Check sheet for the drawn part. Datum: minimum x, y, z corner. Units: mm. A direction names the side the tool comes from. Give positions to 0.01 mm unless a question says otherwise; leave off trailing zeros. Order: outer loops, then holes, each group sorted by start corner. A loop starts at its lowest first (then second) coordinate and runs counter-clockwise, first axis right, second up. Notation, with made-up numbers: M 84.5,16 L 119.5,16 A24 cw 119.5,27 Z; hole C 65,55.5 d11. An arc over 180 degrees is marked long. Answer as CSV lines item,"result". Start each with the question number.
Q1. Set-up check for the marked faces 1 and 2: record each of +Z, -Z, +X, -X, +Y, -Y from which the full face is reachable in a straight line by a thin tool's end or side.
Q2. Section check C-C, the plane z = 3.5. Record the boundary of the cut face in (x, y), then the cut area to 3 significant figures.
Q3. Go/stop test with flat-tipped pins: pin 1 (1.5 mm diameter, centred on y = 5.5, z = 3, fed in from +X); pin 2 (2.5 mm diameter, centred on x = 15, z = 3.5, fed in from -Y). Record where each tip stops, or that it passes through.
Q4. Thickness scan on line 1 (Z direction, x = 0.6, y = 15); line 2 (X direction, y = 8.5, z = 4). Record the ranges inside material, lowest first.
Q5. Section check A-A, the plane x = 15. Record the boundary of the cut face in (y, z).
Q6. Section check D-D, the plane z = 6. Record the boundary of the cut face in (x, y).
Q7. Mould release check, pull along Z, two halves, no side actions. Record for the marked faces 3, 4, 5 and 6: +Z half, -Z half, draft (parallel to the pull), parting line (faces both ways), or undercut.
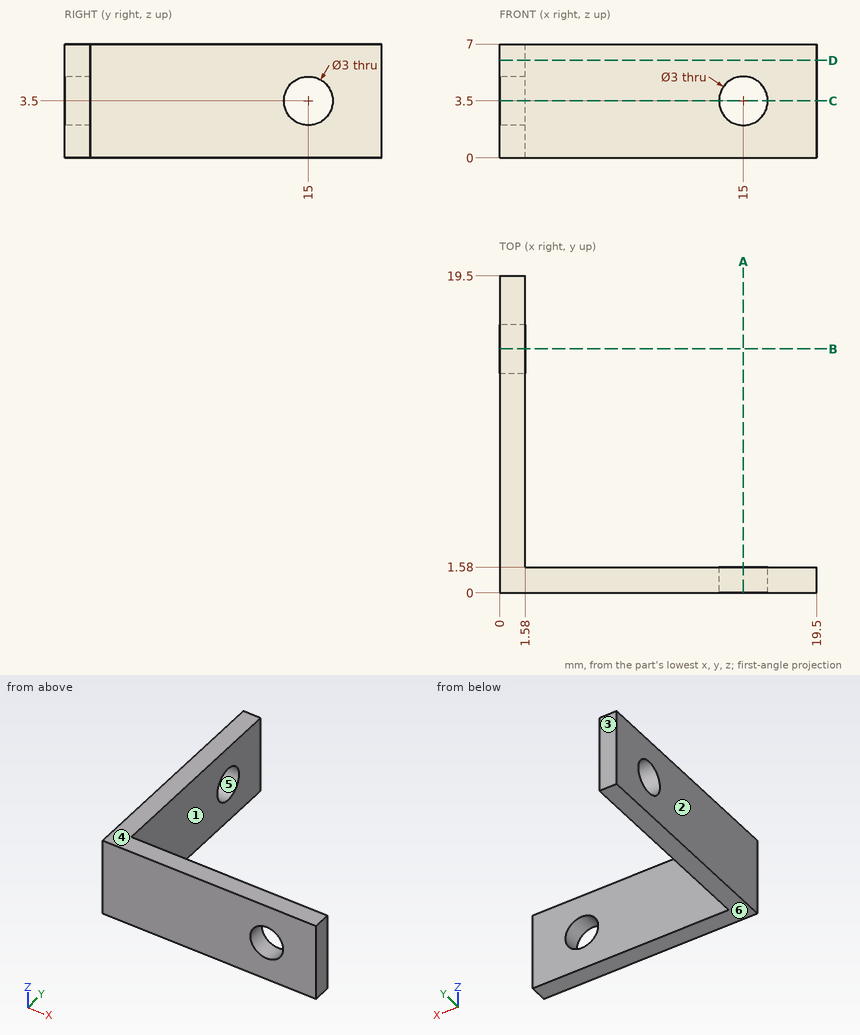
Answer block:
1,face 1,"+Z, -Z, +X, +Y"
1,face 2,"+Z, -Z, -X, +Y, -Y"
2,outline,"M 0,0 L 13.5,0 L 13.5,1.58 L 1.58,1.58 L 1.58,13.5 L 0,13.5 Z; M 0,16.5 L 1.58,16.5 L 1.58,19.5 L 0,19.5 Z; M 16.5,0 L 19.5,0 L 19.5,1.58 L 16.5,1.58 Z"
2,area,"49.6 mm2"
3,pin 1,"stops at x = 1.58"
3,pin 2,"passes through"
4,line 1,"z = 0 to 2, 5 to 7"
4,line 2,"x = 0 to 1.58"
5,outline,"M 0,0 L 1.58,0 L 1.58,2 L 0,2 Z; M 0,5 L 1.58,5 L 1.58,7 L 0,7 Z"
6,outline,"M 0,0 L 19.5,0 L 19.5,1.58 L 1.58,1.58 L 1.58,19.5 L 0,19.5 Z"
7,face 3,"draft"
7,face 4,"+Z half"
7,face 5,"undercut"
7,face 6,"-Z half"
